Here's how the part is built. I have some questions about the finished solid (model axes, mm). A direction names the side the tool comes from. Give positions to 0.01 mm unless a question says otherwise; leave off trailing zeros. Loops run counter-clockwise (first coordinate to the right, second up) from the corner with the lowest first, then second, coordinate; pieces in that order, holes last. Notation, with made-up numbers: (86, -0.5) -> (133, -0.5) arc R25 cw to (133, 26.5) -> close; hole circle Ø6 at (-3.75, -26.75). An arc over 180 degrees is marked (long way). Answer in a Markdown table with one row per item. Add a question column.
Item 1: If we section it at B-B (x = 12): Write out the boundary of the cut face in (y, z).
Item 2: For P1, Ø1.5, axis at x = 19, y = 19, coming from the +Z side; P2, Ø2.5, axis at y = 49, z = 2, coming from the -X side; P3, Ø0.9, axis at x = 18, y = 14, coming from the -Z side, each with a flat end and sliding along its axis, tell me the tip position at first contact or that it passes through.
Item 3: If we section it at D-D (y = 20): Write out the boundary of the cut face in (x, z).
Item 4: If I drill on line 1 (X direction, y = 47.5, z = -3); line 2 (Y direction, x = -6.5, z = 5); line 3 (X direction, y = 20, z = 0), over which ranges is the centre line in solid material (lowest first)?
Item 5: Which directions (+Z, -Z, +X, -X, +Y, -Y) give clear straight access to the entire face, cutting with the end or side of a thin tool? Please do faces 1 (the face through (-16.75, 49, 0)), 2 (the face through (0, 50, 9)), 3 (the face through (19, 36.75, 0)).
Item 6: If we section it at C-C (z = 7.5): Write out the boundary of the cut face in (x, y).
Item 7: We'd pull the mould along Z, two halves only. Please class faces 4 (the face through (19, 20, -8.5)), 5 (the face through (13, 20, -20)), 6 (the face through (13, 20, 20)), 7 (the face through (0, 0, 0)): released by +Z, released by -Z, zero draft, split by the parting line, or undercut.
Item 8: If we section it at A-A (y = 8): Write out the boundary of the cut face in (x, z), then the cut area to 3 significant figures.
```python
from build123d import *

# Parameters (mm, degrees)
CROQUIS1_R              = 20
SALIENTE_EXTRUIR1_DEPTH = 50
CROQUIS3_R              = 20
SALIENTE_EXTRUIR2_DEPTH = 20
CROQUIS4_W              = 33.5
CROQUIS4_H              = 17
CORTAR_EXTRUIR2_DEPTH   = 3
CROQUIS5_W              = 17
CROQUIS5_H              = 33.5
CORTAR_EXTRUIR3_DEPTH   = 3


with BuildPart() as part:
    # Croquis1 → Saliente-Extruir1 (new body)
    with BuildSketch(Plane(origin=(0, 0, 0), x_dir=(1, 0, 0), z_dir=(0, 1, 0))):
        Circle(CROQUIS1_R)
    extrude(amount=SALIENTE_EXTRUIR1_DEPTH)

    # Croquis3 → Saliente-Extruir2 (add)
    with BuildSketch(Plane(origin=(0, 0, 0), x_dir=(0, 0, -1), z_dir=(1, 0, 0))):
        with Locations((0, 20)):
            Circle(CROQUIS3_R)
    extrude(amount=SALIENTE_EXTRUIR2_DEPTH)

    # Croquis4 → Cortar-Extruir2 (cut)
    with BuildSketch(Plane(origin=(0, 50, 0), x_dir=(1, 0, 0), z_dir=(0, 1, 0))):
        Rectangle(CROQUIS4_W, CROQUIS4_H)
    extrude(amount=-CORTAR_EXTRUIR2_DEPTH, mode=Mode.SUBTRACT)

    # Croquis5 → Cortar-Extruir3 (cut)
    with BuildSketch(Plane(origin=(20, 0, 0), x_dir=(0, 0, -1), z_dir=(1, 0, 0))):
        with Locations((0, 20)):
            Rectangle(CROQUIS5_W, CROQUIS5_H)
    extrude(amount=-CORTAR_EXTRUIR3_DEPTH, mode=Mode.SUBTRACT)


solid = part.part
```
Recorded:
| question | item | result |
|---|---|---|
| 1 | outline | (0, -16) -> (8, -16) arc R20 ccw to (32, -16) -> (50, -16) -> (50, -8.5) -> (47, -8.5) -> (47, 8.5) -> (50, 8.5) -> (50, 16) -> (32, 16) arc R20 ccw to (8, 16) -> (0, 16) -> close |
| 2 | P1 | stops at z = 20 |
| 2 | P2 | stops at x = -19.99 |
| 2 | P3 | stops at z = -19.21 |
| 3 | outline | (0, -20) -> (20, -20) -> (20, -8.5) -> (17, -8.5) -> (17, 8.5) -> (20, 8.5) -> (20, 20) -> (0, 20) arc R20 ccw to start |
| 4 | line 1 | x = -19.77 to -16.75, 16.75 to 19.77 |
| 4 | line 2 | y = 0 to 47 |
| 4 | line 3 | x = -20 to 17 |
| 5 | face 1 | +Y |
| 5 | face 2 | +Z, -Z, +X, -X, +Y |
| 5 | face 3 | +X |
| 6 | outline | (-18.54, 0) -> (18.54, 0) -> (18.54, 1.46) -> (20, 1.46) -> (20, 3.25) -> (17, 3.25) -> (17, 36.75) -> (20, 36.75) -> (20, 38.54) -> (18.54, 38.54) -> (18.54, 50) -> (16.75, 50) -> (16.75, 47) -> (-16.75, 47) -> (-16.75, 50) -> (-18.54, 50) -> close |
| 7 | face 4 | undercut |
| 7 | face 5 | released by -Z |
| 7 | face 6 | released by +Z |
| 7 | face 7 | zero draft |
| 8 | outline | (12, -16) -> (20, -16) -> (20, -8.5) -> (17, -8.5) -> (17, 8.5) -> (20, 8.5) -> (20, 16) -> (12, 16) arc R20 ccw (long way) to start |
| 8 | area | 1,280 mm^2 |
